Here's how the part is built. I have some questions about the finished solid (model axes, mm). A direction names the side the tool comes from. Give positions to 0.01 mm unless a question says otherwise; leave off trailing zeros. Write each loop counter-clockwise with the first axis right and the second up, starting at its lowest first coordinate (ties: lowest second). Pieces come first, ordered by that corner, then holes. Notation, with made-up numbers: (-9.5, -7) - (44.5, -7) arc R34 cw to (44.5, 30) - close; hole circle Ø1 at (-19, -28.5). An arc over 180 degrees is marked (long way). One line per item, written item: value. Start each with the question number.
1) Imagine slicing it at C-C on x = 84.5. Write out the boundary of the cut face in (y, z).
2) Imagine slicing it at B-B on z = 5.5. Write out the boundary of the cut face in (x, y).
3) Imagine slicing it at A-A on x = 115. Count the separate pieces of the cut face and the enclosed holes in it, plus the area to 3 significant figures.
4) I'm going to push flat-ended pins straight in: P1, Ø5.5, axis at x = 5, y = 135, coming from the +Z side; P2, Ø1.5, axis at x = 45, y = 5.5, coming from the +Z side; P3, Ø5, axis at y = 45, z = 4.5, coming from the +X side. Where does each tip first touch, or does it pass through?
5) We'd pull the mould along Y, two halves only. Please class faces 4 (the cylindrical face through (115.37, 13.34, -4.77)), 5 (the flat face through (59, 0, -4)), 6 (the flat face through (99, 76, -8)): +Y half, -Y half, draft (parallel to the pull), parting line (faces both ways), or undercut.
6) On a 3-axis mill with a long thin cutter (end or side, diameter ignored), from which of +Z, -Z, +X, -X, +Y, -Y can I reach the whole of each face in a straight line? I mean faces 1 (the cylindrical face through (5.37, 103.34, -4.77)), 2 (the cylindrical face through (58.87, 21.77, -2.03)), 3 (the flat face through (103, 48, 3)). Say none if no direction works.
7) Please list where these lines run through material, in increasing order: L1, parallel to X at y = 145, z = -4.25; L2, parallel to X at y = 130, z = -2.25; L3, parallel to X at y = 15, z = -2.75. Write a range as [from, to].
from build123d import *

# Parameters (mm, degrees)
SKETCH1_W                                     = 120
SKETCH1_H                                     = 150
EXTRUDE1_DEPTH                                = 8
SKETCH2_R                                     = 37.5
EXTRUDE2_DEPTH                                = 9
SKETCH3_R                                     = 7.5
EXTRUDE3_DEPTH                                = 3
SKETCH4_R                                     = 6
EXTRUDE4_DEPTH                                = 10
TAPPED_HOLE1_D                                = 4.2
TAPPED_HOLE1_DEPTH                            = 14
TAPPED_HOLE1_CBORE_D                          = 5
TAPPED_HOLE1_CBORE_DEPTH                      = 10
TAPPED_HOLE1_TIP                              = 1.2618073
SKETCH7_R                                     = 3.5
EXTRUDE5_DEPTH                                = 12
CSK_FOR_FLAT_HEAD_MACHINE_SCREW1_D            = 3.4
CSK_FOR_FLAT_HEAD_MACHINE_SCREW1_CSINK_D      = 6.3
CSK_FOR_FLAT_HEAD_MACHINE_SCREW1_CSINK_ANGLE  = 90
LPATTERN1_COUNT                               = 5
LPATTERN1_PITCH                               = 30
LPATTERN1_COUNT_DIR2                          = 2
LPATTERN1_PITCH_DIR2                          = 110
CBORE_FOR_PAN_HEAD_MACHINE_SCREW2_D           = 2.4
CBORE_FOR_PAN_HEAD_MACHINE_SCREW2_CBORE_D     = 5
CBORE_FOR_PAN_HEAD_MACHINE_SCREW2_CBORE_DEPTH = 1.6
LPATTERN2_COUNT                               = 4
LPATTERN2_PITCH                               = 30
CSK_FOR_FLAT_HEAD_MACHINE_SCREW2_D            = 2.4
CSK_FOR_FLAT_HEAD_MACHINE_SCREW2_CSINK_D      = 4.4
CSK_FOR_FLAT_HEAD_MACHINE_SCREW2_CSINK_ANGLE  = 90
LPATTERN3_COUNT                               = 3
LPATTERN3_PITCH                               = 37.5


with BuildPart() as part:
    # Sketch1 → Extrude1 (new body)
    with BuildSketch(Plane.XY):
        with Locations((60, 75)):
            Rectangle(SKETCH1_W, SKETCH1_H)
    extrude(amount=-EXTRUDE1_DEPTH)

    # Sketch2 → Extrude2 (cut, through all)
    with BuildSketch(Plane.XY):
        with Locations((60, 75)):
            Circle(SKETCH2_R)
    extrude(amount=-EXTRUDE2_DEPTH, mode=Mode.SUBTRACT)

    # Sketch3 → Extrude3 (add)
    with BuildSketch(Plane.XY):
        with Locations((60, 122.5)):
            Circle(SKETCH3_R)
        with Locations((101.13620668, 51.25)):
            Circle(SKETCH3_R)
        with Locations((18.86379332, 51.25)):
            Circle(SKETCH3_R)
    extrude(amount=EXTRUDE3_DEPTH)

    # Sketch4 → Extrude4 (add)
    with BuildSketch(Plane.XY):
        with Locations((22.5, 130)):
            Circle(SKETCH4_R)
        with Locations((97.5, 130)):
            Circle(SKETCH4_R)
        with Locations((60, 20)):
            Circle(SKETCH4_R)
    extrude(amount=EXTRUDE4_DEPTH)

    # Tapped Hole1
    with Locations(Plane.XY.offset(10)):
        with Locations((22.5, 130), (97.5, 130), (60, 20)):
            CounterBoreHole(TAPPED_HOLE1_D / 2, TAPPED_HOLE1_CBORE_D / 2, TAPPED_HOLE1_CBORE_DEPTH, depth=TAPPED_HOLE1_DEPTH)
            with Locations((0, 0, -(TAPPED_HOLE1_DEPTH + TAPPED_HOLE1_TIP / 2))):  # 118° drill point
                Cone(0, TAPPED_HOLE1_D / 2, TAPPED_HOLE1_TIP, mode=Mode.SUBTRACT)

    # Sketch7 → Extrude5 (cut, through all)
    with BuildSketch(Plane.XY.offset(3)):
        with Locations((60, 122.5)):
            Circle(SKETCH7_R)
        with Locations((101.13620668, 51.25)):
            Circle(SKETCH7_R)
        with Locations((18.86379332, 51.25)):
            Circle(SKETCH7_R)
    extrude(amount=-EXTRUDE5_DEPTH, mode=Mode.SUBTRACT)

    # CSK for  Flat Head Machine Screw1 (through all)
    with Locations(Plane.XY):
        with Locations((5, 15)):
            csk_for_flat_head_machine_screw1 = CounterSinkHole(CSK_FOR_FLAT_HEAD_MACHINE_SCREW1_D / 2, CSK_FOR_FLAT_HEAD_MACHINE_SCREW1_CSINK_D / 2, counter_sink_angle=CSK_FOR_FLAT_HEAD_MACHINE_SCREW1_CSINK_ANGLE)

    # LPattern1: CSK for Flat Head Machine Screw1 5 × 2
    with Locations(*[(j * LPATTERN1_PITCH_DIR2, i * LPATTERN1_PITCH, 0) for i in range(LPATTERN1_COUNT) for j in range(LPATTERN1_COUNT_DIR2) if (i, j) != (0, 0)]):
        add(csk_for_flat_head_machine_screw1, mode=Mode.SUBTRACT)

    # CBORE for  Pan Head Machine Screw2 (through all)
    with Locations(Plane.XY):
        with Locations((15, 5)):
            cbore_for_pan_head_machine_screw2 = CounterBoreHole(CBORE_FOR_PAN_HEAD_MACHINE_SCREW2_D / 2, CBORE_FOR_PAN_HEAD_MACHINE_SCREW2_CBORE_D / 2, CBORE_FOR_PAN_HEAD_MACHINE_SCREW2_CBORE_DEPTH)

    # LPattern2: CBORE for  Pan Head Machine Screw2 ×4
    with Locations(*[(i * LPATTERN2_PITCH, 0, 0) for i in range(1, LPATTERN2_COUNT)]):
        add(cbore_for_pan_head_machine_screw2, mode=Mode.SUBTRACT)

    # CSK for  Flat Head Machine Screw2 (through all)
    with Locations(Plane.XY):
        with Locations((22.5, 145)):
            csk_for_flat_head_machine_screw2 = CounterSinkHole(CSK_FOR_FLAT_HEAD_MACHINE_SCREW2_D / 2, CSK_FOR_FLAT_HEAD_MACHINE_SCREW2_CSINK_D / 2, counter_sink_angle=CSK_FOR_FLAT_HEAD_MACHINE_SCREW2_CSINK_ANGLE)

    # LPattern3: CSK for  Flat Head Machine Screw2 ×3
    with Locations(*[(i * LPATTERN3_PITCH, 0, 0) for i in range(1, LPATTERN3_COUNT)]):
        add(csk_for_flat_head_machine_screw2, mode=Mode.SUBTRACT)


solid = part.part
Numbers:
1. outline: (0, -8) - (46.61, -8) - (46.61, 0) - (0, 0) - close; (103.39, -8) - (150, -8) - (150, 0) - (103.39, 0) - close
2. outline: circle Ø12 at (22.5, 130); circle Ø12 at (60, 20); circle Ø12 at (97.5, 130); hole circle Ø5 at (22.5, 130); hole circle Ø5 at (60, 20); hole circle Ø5 at (97.5, 130)
3. separate pieces: 6
3. enclosed holes: 0
3. area: 1,050 mm^2
4. P1: z = -0.4
4. P2: z = -1.6
4. P3: x = 107.32
5. face 4: undercut
5. face 5: -Y half
5. face 6: draft
6. face 1: +Z, -Z
6. face 2: +Z
6. face 3: +Z, +X, -X, -Y
7. L1: [0, 21.3], [23.7, 58.8], [61.2, 96.3], [98.7, 120]
7. L2: [0, 20.4], [24.6, 95.4], [99.6, 120]
7. L3: [0, 3.3], [6.7, 113.3], [116.7, 120]
